Source: CAD feature listing. Evaluate the final solid. Frame: model axes, mm. Face numbers are marked on the shaded views. A direction names the side the tool comes from. Round coordinates to 2 decimals unless told otherwise and drop trailing zeros. Write each loop counter-clockwise with the first axis right and the second up, starting at its lowest first coordinate (ties: lowest second). Pieces come first, ordered by that corner, then holes. Notation, with made-up numbers: M 2,19 L 14,19 A20 ccw 14,30 Z; hole C -39.75,43 d3. An arc over 180 degrees is marked long. Answer in a Markdown table with one row per item.
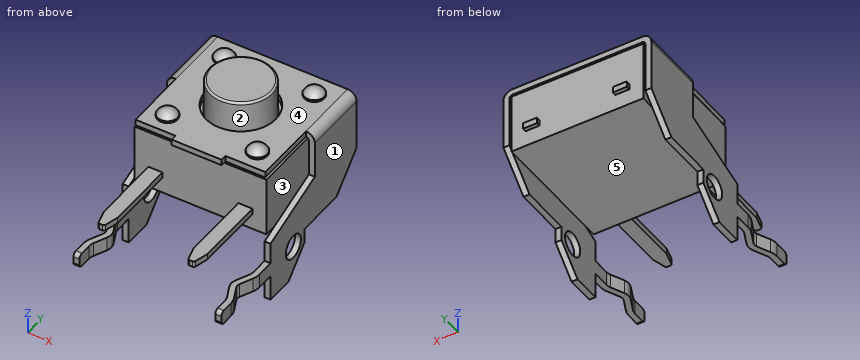
from build123d import *

# Parameters (mm, degrees)
EXTRUDE_THIN1_DEPTH          = 6.8
SKETCH2_R                    = 0.6
CUT_EXTRUDE1_DEPTH           = 13.518086915
CUT_EXTRUDE2_REACH           = 13.606
SKETCH3_R                    = 1.75
EXTRUDE_THIN2_DEPTH          = 0.35
FILLET1_R                    = 0.2
SKETCH6_R                    = 0.5
EXTRUDE1_DEPTH               = 0.1
DOME1_FACE_RADIUS            = 0.5
DOME1_HEIGHT                 = 0.3
LPATTERN1_COUNT              = 2
LPATTERN1_PITCH              = 4.5
LPATTERN1_COUNT_DIR2         = 2
LPATTERN1_PITCH_DIR2         = 4.5
LPATTERN1_COPY_1_FACE_RADIUS = 0.5
LPATTERN1_COPY_1_HEIGHT      = 0.3
LPATTERN1_COPY_2_FACE_RADIUS = 0.5
LPATTERN1_COPY_2_HEIGHT      = 0.3
LPATTERN1_COPY_3_FACE_RADIUS = 0.5
LPATTERN1_COPY_3_HEIGHT      = 0.3
SKETCH7_W                    = 6.6
SKETCH7_H                    = 3
EXTRUDE2_DEPTH               = 6.5
EXTRUDE3_START               = 2.5
SKETCH8_R                    = 1.6
EXTRUDE3_DEPTH               = 3.85
EXTRUDE3_TAPER               = 0.5
FILLET2_R                    = 0.1
EXTRUDE4_DEPTH               = 0.15
FILLET3_R                    = 0.1
FILLET1_OF_MIRROR1_R         = 0.2
FILLET3_OF_MIRROR2_R         = 0.1
EXTRUDE5_REACH               = 13.538
SKETCH10_R                   = 0.4
BODY_MOVE_COPY1_ANGLE        = 180


with BuildPart() as part:
    # Sketch1 → Extrude-Thin1 (new body)
    with BuildSketch(Plane(origin=(0, 2, 0), x_dir=(-1, 0, 0), z_dir=(0, 1, 0))):
        with BuildLine():
            Line((-3.7, 1.65), (-3.7, -4.5))
            ThreePointArc((-3.7, -4.5), (-3.568198052, -4.818198052), (-3.25, -4.95))
            Line((-3.25, -4.95), (3.25, -4.95))
            ThreePointArc((3.25, -4.95), (3.568198052, -4.818198052), (3.7, -4.5))
            Line((3.7, -4.5), (3.7, 1.65))
            Line((3.7, 1.65), (3.4, 1.65))
            Line((3.4, 1.65), (3.4, -4.5))
            ThreePointArc((3.4, -4.5), (3.356066017, -4.606066017), (3.25, -4.65))
            Line((3.25, -4.65), (-3.25, -4.65))
            ThreePointArc((-3.25, -4.65), (-3.356066017, -4.606066017), (-3.4, -4.5))
            Line((-3.4, -4.5), (-3.4, 1.65))
            Line((-3.4, 1.65), (-3.7, 1.65))
        make_face()
    extrude(amount=EXTRUDE_THIN1_DEPTH)

    # Sketch2 → Cut-Extrude1 (cut, through all)
    with BuildSketch(Plane.ZY.offset(3.7)):
        with Locations((0, 3.8)):
            Circle(SKETCH2_R)
        Polygon((-4.65, 2), (-4.65, 5.5), (-2.65, 5.5), (-1.425, 2), align=None)
        Polygon((-1.939540106, 8.8), (-0.35, 7.210459894), (-0.35, 4.682211917), (0.379967393, 4.682211917), (1.65, 3.41217931), (1.65, 8.8), align=None)
    extrude(amount=-CUT_EXTRUDE1_DEPTH, mode=Mode.SUBTRACT)

    # Sketch3 → Cut-Extrude2 (cut, up to next)
    with BuildSketch(Plane(origin=(0, 0, -4.95), x_dir=(-1, 0, 0), z_dir=(0, 0, -1)), mode=Mode.PRIVATE) as cut_extrude2_sk1:
        with Locations((0, 5.5)):
            Circle(SKETCH3_R)
    cut_extrude2_tool1 = extrude(cut_extrude2_sk1.sketch, amount=-CUT_EXTRUDE2_REACH, mode=Mode.PRIVATE) & part.part
    # Sketch3 → Cut-Extrude2 (cut, up to next)
    with BuildSketch(Plane(origin=(0, 0, -4.95), x_dir=(-1, 0, 0), z_dir=(0, 0, -1)), mode=Mode.PRIVATE) as cut_extrude2_sk2:
        Polygon((3.7, 5.5), (3.25, 5.5), (3.25, 2.3), (1.25, 2.3), (1.25, 2), (3.7, 2), align=None)
    cut_extrude2_tool2 = extrude(cut_extrude2_sk2.sketch, amount=-CUT_EXTRUDE2_REACH, mode=Mode.PRIVATE) & part.part
    # Sketch3 → Cut-Extrude2 (cut, up to next)
    with BuildSketch(Plane(origin=(0, 0, -4.95), x_dir=(-1, 0, 0), z_dir=(0, 0, -1)), mode=Mode.PRIVATE) as cut_extrude2_sk3:
        Polygon((-3.7, 5.5), (-3.25, 5.5), (-3.25, 2.3), (-1.25, 2.3), (-1.25, 2), (-3.7, 2), align=None)
    cut_extrude2_tool3 = extrude(cut_extrude2_sk3.sketch, amount=-CUT_EXTRUDE2_REACH, mode=Mode.PRIVATE) & part.part
    add(cut_extrude2_tool1.solids().sort_by_distance((0, 5.5, -4.95))[0], mode=Mode.SUBTRACT)
    add(cut_extrude2_tool2.solids().sort_by_distance((-3.475, 5.457277, -4.95))[0], mode=Mode.SUBTRACT)
    add(cut_extrude2_tool3.solids().sort_by_distance((3.475, 5.457277, -4.95))[0], mode=Mode.SUBTRACT)

    # Sketch5 → Extrude-Thin2 (add, symmetric)
    with BuildSketch(Plane.XY):
        with BuildLine():
            Line((-3.4, 2), (-3.4, 1.131534156))
            ThreePointArc((-3.4, 1.131534156), (-3.386082006, 1.003051153), (-3.344973726, 0.880528901))
            Line((-3.344973726, 0.880528901), (-3.055026274, 0.251005255))
            ThreePointArc((-3.055026274, 0.251005255), (-3, 0), (-3.055026274, -0.251005255))
            Line((-3.055026274, -0.251005255), (-3.344973726, -0.880528901))
            ThreePointArc((-3.344973726, -0.880528901), (-3.386082006, -1.003051153), (-3.4, -1.131534156))
            Line((-3.4, -1.131534156), (-3.4, -1.9))
            Line((-3.4, -1.9), (-3.7, -1.9))
            Line((-3.7, -1.9), (-3.7, -1.131534156))
            ThreePointArc((-3.7, -1.131534156), (-3.679123009, -0.938809651), (-3.617460589, -0.755026274))
            Line((-3.617460589, -0.755026274), (-3.327513137, -0.125502627))
            ThreePointArc((-3.327513137, -0.125502627), (-3.3, 0), (-3.327513137, 0.125502627))
            Line((-3.327513137, 0.125502627), (-3.617460589, 0.755026274))
            ThreePointArc((-3.617460589, 0.755026274), (-3.679123009, 0.938809651), (-3.7, 1.131534156))
            Line((-3.7, 1.131534156), (-3.7, 2))
            Line((-3.7, 2), (-3.4, 2))
        make_face()
    extrude_thin2 = extrude(amount=EXTRUDE_THIN2_DEPTH, both=True)

    # Fillet1
    fillet1_edges = [part.edges().sort_by_distance(p)[0] for p in [
        (-3.55, -1.9, 0.35),
        (-3.55, -1.9, -0.35),
    ]]
    fillet(fillet1_edges, radius=FILLET1_R)

    # Sketch6 → Extrude1 (add)
    with BuildSketch(Plane(origin=(0, 0, -4.95), x_dir=(-1, 0, 0), z_dir=(0, 0, -1))):
        with Locations(Location((-2.25, 3.25, 0), (0, 0, 180))):
            Circle(SKETCH6_R)
    extrude1 = extrude(amount=EXTRUDE1_DEPTH)

    # Dome1: a dome of height H over a round flat face of radius A is a cap of a sphere of radius (A * A + H * H) / (2 * H)
    dome1_r = (DOME1_FACE_RADIUS * DOME1_FACE_RADIUS + DOME1_HEIGHT * DOME1_HEIGHT) / (2 * DOME1_HEIGHT)
    dome1_base = Plane((2.25, 3.25, -5.05), z_dir=(0, 0, -1))
    with Locations(dome1_base.offset(DOME1_HEIGHT - dome1_r)):
        dome1_ball = Sphere(dome1_r, mode=Mode.PRIVATE)
    add(split(dome1_ball, bisect_by=dome1_base, keep=Keep.TOP, mode=Mode.PRIVATE))

    # LPattern1: Extrude1 2 × 2
    with Locations(*[(-j * LPATTERN1_PITCH_DIR2, i * LPATTERN1_PITCH, 0) for i in range(LPATTERN1_COUNT) for j in range(LPATTERN1_COUNT_DIR2) if (i, j) != (0, 0)]):
        add(extrude1)

    # LPattern1 copy 1: a dome of height H over a round flat face of radius A is a cap of a sphere of radius (A * A + H * H) / (2 * H)
    lpattern1_copy_1_r = (LPATTERN1_COPY_1_FACE_RADIUS * LPATTERN1_COPY_1_FACE_RADIUS + LPATTERN1_COPY_1_HEIGHT * LPATTERN1_COPY_1_HEIGHT) / (2 * LPATTERN1_COPY_1_HEIGHT)
    lpattern1_copy_1_base = Plane((-2.25, 3.25, -5.05), z_dir=(0, 0, -1))
    with Locations(lpattern1_copy_1_base.offset(LPATTERN1_COPY_1_HEIGHT - lpattern1_copy_1_r)):
        lpattern1_copy_1_ball = Sphere(lpattern1_copy_1_r, mode=Mode.PRIVATE)
    add(split(lpattern1_copy_1_ball, bisect_by=lpattern1_copy_1_base, keep=Keep.TOP, mode=Mode.PRIVATE))

    # LPattern1 copy 2: a dome of height H over a round flat face of radius A is a cap of a sphere of radius (A * A + H * H) / (2 * H)
    lpattern1_copy_2_r = (LPATTERN1_COPY_2_FACE_RADIUS * LPATTERN1_COPY_2_FACE_RADIUS + LPATTERN1_COPY_2_HEIGHT * LPATTERN1_COPY_2_HEIGHT) / (2 * LPATTERN1_COPY_2_HEIGHT)
    lpattern1_copy_2_base = Plane((2.25, 7.75, -5.05), z_dir=(0, 0, -1))
    with Locations(lpattern1_copy_2_base.offset(LPATTERN1_COPY_2_HEIGHT - lpattern1_copy_2_r)):
        lpattern1_copy_2_ball = Sphere(lpattern1_copy_2_r, mode=Mode.PRIVATE)
    add(split(lpattern1_copy_2_ball, bisect_by=lpattern1_copy_2_base, keep=Keep.TOP, mode=Mode.PRIVATE))

    # LPattern1 copy 3: a dome of height H over a round flat face of radius A is a cap of a sphere of radius (A * A + H * H) / (2 * H)
    lpattern1_copy_3_r = (LPATTERN1_COPY_3_FACE_RADIUS * LPATTERN1_COPY_3_FACE_RADIUS + LPATTERN1_COPY_3_HEIGHT * LPATTERN1_COPY_3_HEIGHT) / (2 * LPATTERN1_COPY_3_HEIGHT)
    lpattern1_copy_3_base = Plane((-2.25, 7.75, -5.05), z_dir=(0, 0, -1))
    with Locations(lpattern1_copy_3_base.offset(LPATTERN1_COPY_3_HEIGHT - lpattern1_copy_3_r)):
        lpattern1_copy_3_ball = Sphere(lpattern1_copy_3_r, mode=Mode.PRIVATE)
    add(split(lpattern1_copy_3_ball, bisect_by=lpattern1_copy_3_base, keep=Keep.TOP, mode=Mode.PRIVATE))

    # Mirror1: Extrude-Thin2 across plane
    add(extrude_thin2.mirror(Plane(origin=(0, 0, 0), x_dir=(0, 0, 1), z_dir=(1, 0, 0))))

    # Fillet1 of Mirror1
    fillet1_of_mirror1_edges = [part.edges().sort_by_distance(p)[0] for p in [
        (3.55, -1.9, 0.35),
        (3.55, -1.9, -0.35),
    ]]
    fillet(fillet1_of_mirror1_edges, radius=FILLET1_OF_MIRROR1_R)

    # Sketch10 → Extrude5 (add, up to next)
    with BuildSketch(Plane(origin=(0, 0, -4.55), x_dir=(-1, 0, 0), z_dir=(0, 0, -1)), mode=Mode.PRIVATE) as extrude5_sk1:
        with Locations(Location((-2.25, 7.75, 0), (0, 0, 180))):
            Circle(SKETCH10_R)
    extrude5_tool1 = extrude(extrude5_sk1.sketch, amount=EXTRUDE5_REACH, mode=Mode.PRIVATE) - part.part
    # Sketch10 → Extrude5 (add, up to next)
    with BuildSketch(Plane(origin=(0, 0, -4.55), x_dir=(-1, 0, 0), z_dir=(0, 0, -1)), mode=Mode.PRIVATE) as extrude5_sk2:
        with Locations(Location((2.25, 7.75, 0), (0, 0, 180))):
            Circle(SKETCH10_R)
    extrude5_tool2 = extrude(extrude5_sk2.sketch, amount=EXTRUDE5_REACH, mode=Mode.PRIVATE) - part.part
    # Sketch10 → Extrude5 (add, up to next)
    with BuildSketch(Plane(origin=(0, 0, -4.55), x_dir=(-1, 0, 0), z_dir=(0, 0, -1)), mode=Mode.PRIVATE) as extrude5_sk3:
        with Locations(Location((-2.25, 3.25, 0), (0, 0, 180))):
            Circle(SKETCH10_R)
    extrude5_tool3 = extrude(extrude5_sk3.sketch, amount=EXTRUDE5_REACH, mode=Mode.PRIVATE) - part.part
    # Sketch10 → Extrude5 (add, up to next)
    with BuildSketch(Plane(origin=(0, 0, -4.55), x_dir=(-1, 0, 0), z_dir=(0, 0, -1)), mode=Mode.PRIVATE) as extrude5_sk4:
        with Locations(Location((2.25, 3.25, 0), (0, 0, 180))):
            Circle(SKETCH10_R)
    extrude5_tool4 = extrude(extrude5_sk4.sketch, amount=EXTRUDE5_REACH, mode=Mode.PRIVATE) - part.part


with BuildPart() as body_2:
    # Sketch7 → Extrude2 (new body)
    with BuildSketch(Plane(origin=(0, 8.8, 0), x_dir=(-1, 0, 0), z_dir=(0, 1, 0))):
        with Locations((0, -3.05)):
            Rectangle(SKETCH7_W, SKETCH7_H)
    extrude(amount=-EXTRUDE2_DEPTH)

    # Sketch8 → Extrude3 (add)
    with BuildSketch(Plane(origin=(0, 0, 0), x_dir=(-1, 0, 0), z_dir=(0, 0, -1)).offset(EXTRUDE3_START)):
        with Locations((0, 5.5)):
            Circle(SKETCH8_R)
    extrude(amount=EXTRUDE3_DEPTH, taper=EXTRUDE3_TAPER)

    # Fillet2
    fillet2_edges = [body_2.edges().sort_by_distance(p)[0] for p in [
        (1.566401559, 5.5, -6.35),
    ]]
    fillet(fillet2_edges, radius=FILLET2_R)

    # Sketch9 → Extrude4 (add, symmetric)
    with BuildSketch(Plane(origin=(0, 0, -2.5), x_dir=(-1, 0, 0), z_dir=(0, 0, -1))):
        Polygon((2.6, 9), (1.9, 9), (1.9, -1.25), (2.100961894, -2), (2.399038106, -2), (2.6, -1.25), align=None)
    extrude4 = extrude(amount=EXTRUDE4_DEPTH, both=True)

    # Fillet3
    fillet3_edges = [body_2.edges().sort_by_distance(p)[0] for p in [
        (-2.100961894, -2, -2.5),
        (-2.399038106, -2, -2.5),
    ]]
    fillet(fillet3_edges, radius=FILLET3_R)

    # Mirror2: Extrude4 across plane
    add(extrude4.mirror(Plane(origin=(0, 0, 0), x_dir=(0, 0, 1), z_dir=(1, 0, 0))))

    # Fillet3 of Mirror2
    fillet3_of_mirror2_edges = [body_2.edges().sort_by_distance(p)[0] for p in [
        (2.100961894, -2, -2.5),
        (2.399038106, -2, -2.5),
    ]]
    fillet(fillet3_of_mirror2_edges, radius=FILLET3_OF_MIRROR2_R)


with BuildPart() as part_1:
    add(part.part)

    add(body_2.part)  # Extrude5 merges body 2
    add(extrude5_tool1.solids().sort_by_distance((2.25, 7.75, -4.55))[0])
    add(extrude5_tool2.solids().sort_by_distance((-2.25, 7.75, -4.55))[0])
    add(extrude5_tool3.solids().sort_by_distance((2.25, 3.25, -4.55))[0])
    add(extrude5_tool4.solids().sort_by_distance((-2.25, 3.25, -4.55))[0])


with BuildPart() as part_2:
    # Body-Move_Copy1: moved
    add(part_1.part.rotate(Axis((0, 0, 0), (0, 1, 0)), BODY_MOVE_COPY1_ANGLE))


with BuildPart() as part_3:
    # Body-Move_Copy2: moved
    add(part_2.part.moved(Location((0, -2, 0))))


solid = part_3.part
Q1. Section B-B (z = 0). State how many separate pieces and enclosed holes the cut face has, and give its area (3 significant figures).
Solutions:
| item | result |
|---|---|
| separate pieces | 4 |
| enclosed holes | 0 |
| area | 3.32 mm2 |
Q2. Pull-direction query (Y, two-part tool) for the marked faces 4 and 5; classes: pulls with the +Y half, pulls with the -Y half, needs draft (parallel to the pull), parting line crosses it, or undercut.
Solutions:
| item | result |
|---|---|
| face 4 | undercut |
| face 5 | needs draft |
Q3. Access query for the marked faces 1, 2 and 3. Directions: +Z, -Z, +X, -X, +Y, -Y. A direction counts if a zero-diameter tool reaches every point of the face in a straight line with its end or side. Return the directions, or none.
Solutions:
| item | result |
|---|---|
| face 1 | +Z, -Z, +X, +Y, -Y |
| face 2 | +Z |
| face 3 | -Z, +Y, -Y |
Q4. Section D-D (z = 6). Return loops of the section in (x, y).
Solutions:
| item | result |
|---|---|
| outline | C 0,3.5 d3.14 |
Q5. Material intervals for probe 1 along Y at (x, z) = (0, 4.85); probe 2 along X at (y, z) = (5.75, 1.5); probe 3 along X at (y, z) = (3.25, 4.25), sorted ascending.
Solutions:
| item | result |
|---|---|
| probe 1 | y = 0 to 1.75, 1.92 to 5.08, 5.25 to 6.8 |
| probe 2 | x = -3.7 to -3.4, 3.4 to 3.7 |
| probe 3 | x = -3.3 to 3.3 |
Q6. Contact query for flat-ended pins moving along their axis: pin 1 Ø1 at (x, y) = (-2.5, 5) entering from +Z; pin 2 Ø3 at (x, y) = (-0.5, 4.5) entering from -Z; pin 3 Ø0.8 at (x, y) = (2.5, -1) entering from +Z. Output: stop coordinate, or through.
Solutions:
| item | result |
|---|---|
| pin 1 | stops at z = 5.27 |
| pin 2 | stops at z = 1.55 |
| pin 3 | stops at z = 2.65 |
